```python
from build123d import *

# Parameters (mm, degrees)
F0_R     = 212.5
F1_DEPTH = 8
F2_R     = 3.25
F3_DEPTH = 5


with BuildPart() as f1:
    # F0 (on Top) → F1 (new body)
    with BuildSketch(Plane.XY):
        Circle(F0_R)
    extrude(amount=F1_DEPTH)

    # F2 (on face) → F3 (join)
    with BuildSketch(Plane(origin=(0, 0, 0), x_dir=(1, 0, 0), z_dir=(0, 0, -1))):
        with Locations((0, 207.5)):
            Circle(F2_R)
        with Locations((-179.700271, -103.75)):
            Circle(F2_R)
        with Locations((179.700271, -103.75)):
            Circle(F2_R)
    extrude(amount=F3_DEPTH)


solid = f1.part
```
Read the model definition and answer for the solid it produces. Units are mm, in the model's axes. Round coordinates to 2 decimals unless told otherwise and drop trailing zeros. Loops run counter-clockwise (first coordinate to the right, second up) from the corner with the lowest first, then second, coordinate; pieces in that order, holes last. Notation, with made-up numbers: (-36.75, 76) -> (20.25, 76) arc R19 cw to (20.25, 94) -> close; hole circle Ø9 at (88.5, 62). An arc over 180 degrees is marked (long way). One line per item, written item: value.
1) A cutting plane is placed at C-C (x = 106). Determine the outline of the cut face in (y, z), and give its area (3 significant figures).
Answer list:
outline: (-184.17, 0) -> (184.17, 0) -> (184.17, 8) -> (-184.17, 8) -> close
area: 2,950 mm²
2) A cutting plane is placed at A-A (z = -2.75). Determine the outline of the cut face in (x, y).
Answer list:
outline: circle Ø6.5 at (-179.7, 103.75); circle Ø6.5 at (0, -207.5); circle Ø6.5 at (179.7, 103.75)
3) Flat-ended cylindrical pins translate along their axes: P1, Ø3, axis at y = 131, z = 5, coming from the +X side; P2, Ø2, axis at x = 43.5, z = 6.5, coming from the -Y side; P3, Ø1, axis at y = 145, z = -2, coming from the -X side; P4, Ø6, axis at x = -121, y = 92.5, coming from the -Z side. Find the tip coordinate at first contact, or state that the pin passes through.
Answer list:
P1: stops at x = 168.48
P2: stops at y = -208.21
P3: passes through
P4: stops at z = 0
4) A cutting plane is placed at B-B (y = 0). Determine the outline of the cut face in (x, z), and give its area (3 significant figures).
Answer list:
outline: (-212.5, 0) -> (212.5, 0) -> (212.5, 8) -> (-212.5, 8) -> close
area: 3,400 mm²
5) Consider L1, parallel to Z at x = -53, y = -115.5; L2, parallel to Y at x = -163, z = 2.75; L3, parallel to Y at x = -187, z = 1. Determine where each line is inside the solid, lowest interval first. Write a range as [from, to].
Answer list:
L1: z = [0, 8]
L2: y = [-136.34, 136.34]
L3: y = [-100.93, 100.93]
